Geometry check sheet. Reference: drawing and pictorial views, mm from the part's lowest x, y, z. A direction names the side the tool comes from. Give positions to 0.01 mm unless a question says otherwise; leave off trailing zeros. Loops run counter-clockwise (first coordinate to the right, second up) from the corner with the lowest first, then second, coordinate; pieces in that order, holes last. Notation, with made-up numbers: M 33,-35.5 L 65,-35.5 A15 ccw 65,-11.5 Z; hole C -7.75,52 d6. An arc over 180 degrees is marked long. One line per question, with ' | ' between items. Start each with the question number.
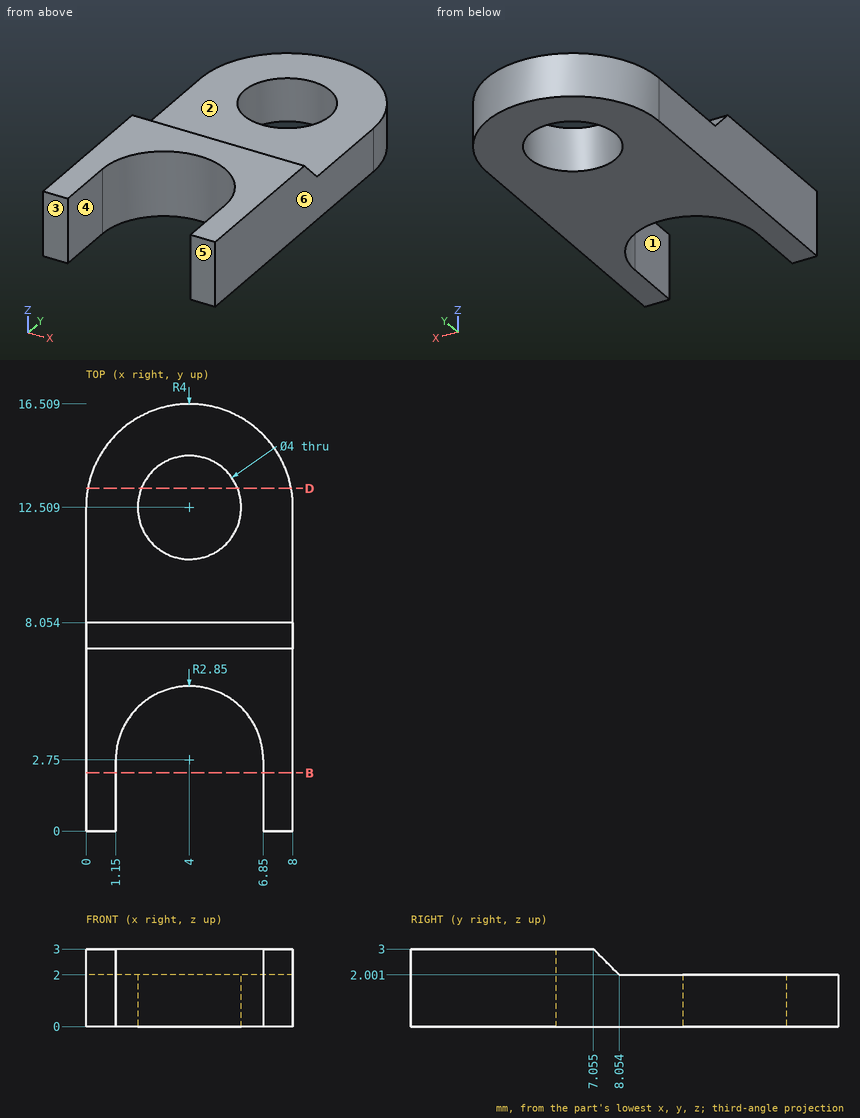
Q1. Access from +Z, -Z, +X, -X, +Y, -Y to the whole of each face (thin tool, end or side, straight path). Record for the marked faces 1, 2 and 3.
Q2. Depth check by flat-ended pin: P1, Ø4, axis at x = 4, y = 13, coming from the +Z side. Enter the tip coordinate at first touch or a pass-through.
Q3. Cross-section at D-D (y = 13.25). Record the cut outline in (x, z).
Q4. Material ranges on probe 1 along Z at (x, y) = (0.5, 10); probe 2 along Y at (x, z) = (4, 0.65); probe 3 along X at (y, z) = (3.25, 0.25) (1 decimal), recorded low to high. Write a range as from..to.
Q5. Draft check along X on the marked faces 4, 5 and 6. Enter one of: released by +X, released by -X, zero draft, split by the parting line, or undercut.
Q6. Cross-section at B-B (y = 2.25). Record the cut outline in (x, z).
Solved:
1) face 1: +Z, -Z, -Y | face 2: +Z, +X, -X, +Y | face 3: +Z, -Z, +X, -X, -Y
2) P1: stops at z = 2
3) outline: M 0.07,0 L 2.14,0 L 2.14,2 L 0.07,2 Z; M 5.86,0 L 7.93,0 L 7.93,2 L 5.86,2 Z
4) probe 1: z = 0..2 | probe 2: y = 5.6..10.51, 14.51..16.51 | probe 3: x = 0..1.2, 6.8..8
5) face 4: undercut | face 5: zero draft | face 6: released by +X
6) outline: M 0,0 L 1.15,0 L 1.15,3 L 0,3 Z; M 6.85,0 L 8,0 L 8,3 L 6.85,3 Z
